Input: part model. Units: mm. Frame: model coordinates. A direction names the side the tool comes from. Coordinates: 2 decimals unless noted, no trailing zeros. Write each loop counter-clockwise with the first axis right and the second up, starting at its lowest first coordinate (ties: lowest second). Pieces come first, ordered by that corner, then holes. Notation, with made-up numbers: M 63.5,-29.5 L 80.5,-29.5 A26 ccw 80.5,-13.5 Z; hole C 61,84 d1. An arc over 180 degrees is marked long. Use one line per item in the form item = value.
from build123d import *

# Parameters (mm, degrees)
SKETCH1_R           = 36.5125
BOSS_EXTRUDE1_DEPTH = 10.16
SKETCH2_R           = 28.8925
SKETCH2_R_2         = 10.16
CUT_EXTRUDE1_DEPTH  = 3.175
SKETCH3_R           = 28.8925
SKETCH3_R_2         = 10.16
CUT_EXTRUDE2_DEPTH  = 3.175
SKETCH4_R           = 10.16
CUT_EXTRUDE3_DEPTH  = 1.27
SKETCH7_R           = 10.16
CUT_EXTRUDE5_DEPTH  = 1.27
FILLET1_R           = 1.27


with BuildPart() as part:
    # Sketch1 → Boss-Extrude1 (new body)
    with BuildSketch(Plane.XY):
        Circle(SKETCH1_R)
        Polygon((3.569234353, -6.4049902), (7.331501401, -0.111447478), (3.762267048, 6.293542722), (-3.569234353, 6.4049902), (-7.331501401, 0.111447478), (-3.762267048, -6.293542722), align=None, mode=Mode.SUBTRACT)
    extrude(amount=BOSS_EXTRUDE1_DEPTH)

    # Sketch2 → Cut-Extrude1 (cut)
    with BuildSketch(Plane.XY.offset(10.16)):
        Circle(SKETCH2_R)
        Circle(SKETCH2_R_2, mode=Mode.SUBTRACT)
    extrude(amount=-CUT_EXTRUDE1_DEPTH, mode=Mode.SUBTRACT)

    # Sketch3 → Cut-Extrude2 (cut)
    with BuildSketch(Plane(origin=(0, 0, 0), x_dir=(-1, 0, 0), z_dir=(0, 0, -1))):
        Circle(SKETCH3_R)
        Circle(SKETCH3_R_2, mode=Mode.SUBTRACT)
    extrude(amount=-CUT_EXTRUDE2_DEPTH, mode=Mode.SUBTRACT)

    # Sketch4 → Cut-Extrude3 (cut)
    with BuildSketch(Plane(origin=(0, 0, 0), x_dir=(-1, 0, 0), z_dir=(0, 0, -1))):
        Circle(SKETCH4_R)
    extrude(amount=-CUT_EXTRUDE3_DEPTH, mode=Mode.SUBTRACT)

    # Sketch7 → Cut-Extrude5 (cut)
    with BuildSketch(Plane.XY.offset(10.16)):
        Circle(SKETCH7_R)
    extrude(amount=-CUT_EXTRUDE5_DEPTH, mode=Mode.SUBTRACT)

    # Fillet1
    fillet1_edges = [part.edges().sort_by_distance(p)[0] for p in [
        (-28.8925, 0, 6.985),
        (-10.16, 0, 6.985),
        (28.8925, 0, 3.175),
        (10.16, 0, 3.175),
    ]]
    fillet(fillet1_edges, radius=FILLET1_R)


solid = part.part
(1) Section query A-A on z = 5.5. Return the cut outline in (x, y) (1 decimal), plus the area to 3 significant figures.
Computed:
outline = C 0,0 d73; hole M -7.3,0.1 L -3.8,-6.3 L 3.6,-6.4 L 7.3,-0.1 L 3.8,6.3 L -3.6,6.4 Z
area = 4,050 mm^2
(2) Pull-direction query (X, two-part tool) for faces 1 (the flat face through (27, 11, 0)), 2 (the cylindrical face through (34.826, 10.967, 5.009)), 3 (the cylindrical face through (-1.323, 10.074, 8.577)); classes: pulls with the +X half, pulls with the -X half, needs draft (parallel to the pull), parting line crosses it, or undercut.
Computed:
face_1 = needs draft
face_2 = parting line crosses it
face_3 = undercut
(3) Line query: probe 1 along Y at (x, z) = (0, 1.35); probe 2 along Y at (x, z) = (0, 0.95); probe 3 along Z at (x, y) = (12, 21) (3 decimals). Output: solid intervals per line, ascending.
Computed:
probe_1 = -36.51 to -28.89, -10.16 to -6.35, 6.35 to 10.16, 28.89 to 36.51
probe_2 = -36.51 to -28.89, 28.89 to 36.51
probe_3 = 3.175 to 6.985
(4) Set-up query: faces 4 (the cylindrical face through (1.323, 10.074, 1.583)), 5 (the flat face through (-5.424, 3.302, 5.027)), 6 (the flat face through (0, -7, 8.89)). Return all of +Z, -Z, +X, -X, +Y, -Y with unobstructed straight access to the full face (end or side cutting, diameter ignored); none if empty.
Computed:
face_4 = -Z
face_5 = +Z, -Z
face_6 = +Z
(5) First-contact query: pin 1 Ø16.5 at (x, y) = (-4, 9) entering from -Z; pin 2 Ø6 at (x, y) = (-19, -12.5) entering from +Z (3 decimals); pin 3 Ø1 at (y, z) = (-20.5, 1.5) entering from -X. Flat tips, straight axial feed; report the tip coordinate or a pass-through.
Computed:
pin_1 = 1.27
pin_2 = 6.985
pin_3 = -30.55
